from build123d import *

# Parameters (mm, degrees)
F1_DEPTH  = 85
F2_R      = 10
F4_DEPTH  = 6
F5_R      = 2
F6_W      = 7.7781745931
F6_H      = 15
F7_DEPTH  = 6
F8_R      = 2
F6_R      = 1.1
F9_DEPTH  = 1.5
F3_R      = 1.1
F10_DEPTH = 1.5
F11_W     = 18.7703792453
F11_H     = 83
F12_DEPTH = 8


with BuildPart() as f1:
    # F0 (on Top) → F1 (new body)
    with BuildSketch(Plane.XY):
        Polygon((-20, 20), (-14.5, 14.5), (-10.3851896226, 18.6148103774), (0, 18.6148103774), (10.3851896226, 18.6148103774), (14.5, 14.5), (20, 20), (12.470660899, 27.529339101), (0, 27.529339101), (-12.470660899, 27.529339101), align=None)
    extrude(amount=F1_DEPTH)

    # F2
    f2_edges = [f1.edges().sort_by_distance(p)[0] for p in [
        (-12.470661, 27.529339, 42.5),
        (12.470661, 27.529339, 42.5),
    ]]
    fillet(f2_edges, radius=F2_R)

    # F3 (on face) → F4 (cut)
    with BuildSketch(Plane(origin=(0, 0, 0), x_dir=(0.7071067812, 0.7071067812, 0), z_dir=(0.7071067812, -0.7071067812, 0))):
        Polygon((28.2842712475, 59.0200200677), (28.2842712475, 74.0199925453), (20.5060966544, 74.0199925453), (20.5060966544, 0), (20.6173848753, 0), (20.6173848753, 9.0200751125), (28.2842712475, 9.0200751125), (28.2842712475, 24.0200475901), (20.5802888017, 24.0200475901), (20.5802888017, 34.0200475901), (28.2842712475, 34.0200475901), (28.2842712475, 49.0200200677), (20.543192728, 49.0200200677), (20.543192728, 59.0200200677), align=None)
    extrude(amount=-F4_DEPTH, mode=Mode.SUBTRACT)

    # F5
    f5_edges = [f1.edges().sort_by_distance(p)[0] for p in [
        (17.87868, 22.12132, 74.019993),
        (17.87868, 22.12132, 49.02002),
        (17.87868, 22.12132, 24.020048),
        (17.699797, 22.300203, 0),
        (12.457372, 16.700013, 0),
        (12.431141, 16.673782, 24.020048),
        (12.404911, 16.647551, 49.02002),
        (17.699797, 22.300203, 85),
        (12.442595, 16.557405, 85),
        (17.87868, 22.12132, 59.02002),
        (12.404911, 16.647551, 59.02002),
        (17.87868, 22.12132, 34.020048),
        (12.431141, 16.673782, 34.020048),
        (17.87868, 22.12132, 9.020075),
        (12.457372, 16.700013, 9.020075),
        (-17.699797, 22.300203, 0),
        (-17.699797, 22.300203, 85),
        (-12.15536, 26.768134, 0),
        (0, 27.529339, 0),
        (12.15536, 26.768134, 0),
        (-12.442595, 16.557405, 0),
        (-12.15536, 26.768134, 85),
        (0, 27.529339, 85),
        (-12.442595, 16.557405, 85),
        (12.15536, 26.768134, 85),
        (12.442595, 16.557405, 74.019993),
    ]]
    fillet(f5_edges, radius=F5_R)

    # F6 (on face) → F7 (cut)
    with BuildSketch(Plane(origin=(0, 0, 0), x_dir=(0.7071067812, -0.7071067812, 0), z_dir=(-0.7071067812, -0.7071067812, 0))):
        with Locations((-24.3951839509, 17.5)):
            Rectangle(F6_W, F6_H)
        with Locations((-24.3951839509, 42.5)):
            Rectangle(F6_W, F6_H)
        with Locations((-24.3951839509, 67.5)):
            Rectangle(F6_W, F6_H)
    extrude(amount=-F7_DEPTH, mode=Mode.SUBTRACT)

    # F8
    f8_edges = [f1.edges().sort_by_distance(p)[0] for p in [
        (-17.87868, 22.12132, 35),
        (-17.87868, 22.12132, 50),
        (-17.87868, 22.12132, 60),
        (-17.87868, 22.12132, 75),
        (-12.442595, 16.557405, 75),
        (-12.442595, 16.557405, 60),
        (-12.442595, 16.557405, 50),
        (-12.442595, 16.557405, 35),
        (-12.442595, 16.557405, 25),
        (-12.442595, 16.557405, 10),
        (-17.87868, 22.12132, 10),
        (-17.87868, 22.12132, 25),
    ]]
    fillet(f8_edges, radius=F8_R)

    # F6 (on face) → F9 (join)
    with BuildSketch(Plane(origin=(0, 0, 0), x_dir=(0.7071067812, -0.7071067812, 0), z_dir=(-0.7071067812, -0.7071067812, 0))):
        with Locations((-24.3951839509, 5)):
            Circle(F6_R)
        with Locations((-24.3951839509, 30)):
            Circle(F6_R)
        with Locations((-24.3951839509, 55)):
            Circle(F6_R)
        with Locations((-24.3951839509, 80)):
            Circle(F6_R)
    extrude(amount=F9_DEPTH)

    # F3 (on face) → F10 (join)
    with BuildSketch(Plane(origin=(0, 0, 0), x_dir=(0.7071067812, 0.7071067812, 0), z_dir=(0.7071067812, -0.7071067812, 0))):
        with Locations((24.3951839509, 79.0199925453)):
            Circle(F3_R)
        with Locations((24.4336626312, 54.0200221575)):
            Circle(F3_R)
        with Locations((24.4721413114, 29.0200517697)):
            Circle(F3_R)
        with Locations((24.5106199916, 4.0200813819)):
            Circle(F3_R)
    extrude(amount=F10_DEPTH)

    # F11 (on face) → F12 (cut)
    with BuildSketch(Plane.XZ.offset(-18.6148103774)):
        with Locations((0, 42.5)):
            Rectangle(F11_W, F11_H)
    extrude(amount=-F12_DEPTH, mode=Mode.SUBTRACT)


solid = f1.part
Source: CAD feature listing. Evaluate the final solid. Frame: model axes, mm. A direction names the side the tool comes from. Round coordinates to 2 decimals unless told otherwise and drop trailing zeros. Order: outer loops, then holes, each group sorted by start corner. A loop starts at its lowest first (then second) coordinate and runs counter-clockwise, first axis right, second up. Notation, with made-up numbers: (-10.75, 26) -> (20.25, 26) arc R16 cw to (20.25, 34) -> close; hole circle Ø10 at (-13.75, 15.25). An arc over 180 degrees is marked (long way). Answer as CSV lines item,"result".
Item 1: Reachability of faces 1 (the face through (-12.84, 17.01, 84.43)), 2 (the face through (15, 19, 9.02)), 3 (the face through (-17.446, 21.748, 9.399)), 4 (the face through (-12.82, 16.99, 75.6)), 5 (the face through (-12, 17, 5)) from +Z, -Z, +X, -X, +Y, -Y: full face, straight path, thin tool, end or side. Return the list, or none.
A:
face 1,"+Z, -Y"
face 2,"+X, -Y"
face 3,"-X"
face 4,"-Y"
face 5,"+Z, -Z, -Y"
Item 2: Section A-A, the plane z = 44. Return loops of the section in (x, y).
A:
outline,"(-15.76, 24.24) -> (-10.26, 18.74) -> (-10.39, 18.61) -> (-9.39, 18.61) -> (-9.39, 26.61) -> (9.39, 26.61) -> (9.39, 18.61) -> (10.39, 18.61) -> (10.26, 18.74) -> (15.76, 24.24) -> (15.4, 24.6) arc R10 ccw to (8.33, 27.53) -> (-8.33, 27.53) arc R10 ccw to (-15.4, 24.6) -> close"
Item 3: Pull-direction query (X, two-part tool) for faces 6 (the face through (-17.446, 21.748, 75.601)), 7 (the face through (12.827, 17.129, 33.45)), 8 (the face through (0, 27.529, 42)); classes: pulls with the +X half, pulls with the -X half, needs draft (parallel to the pull), parting line crosses it, or undercut.
A:
face 6,"pulls with the -X half"
face 7,"undercut"
face 8,"needs draft"
Item 4: Section B-B, the plane x = -7.5. Return loops of the section in (y, z), plus the area to 3 significant figures.
A:
outline,"(18.61, 0) -> (25.53, 0) arc R2 ccw to (27.53, 2) -> (27.53, 83) arc R2 ccw to (25.53, 85) -> (18.61, 85) -> (18.61, 84) -> (26.61, 84) -> (26.61, 1) -> (18.61, 1) -> close"
area,"92.0 mm²"
Item 5: Line query: L1, parallel to X at y = 18.75, z = 13; L2, parallel to Z at x = 15, y = 16.25; L3, parallel to Z at x = -6, y = 23. Output: solid intervals per line, ascending.
A:
L1,"-10.26 to -9.39, 9.39 to 10.26"
L2,"0.07 to 8.95, 24.08 to 33.96, 49.07 to 58.97, 74.06 to 84.96"
L3,"0 to 1, 84 to 85"
Item 6: Pin query (flat end, axial travel): pin 1 Ø4 at (x, y) = (2, 18.5) entering from +Z; pin 2 Ø4 at (y, z) = (24, 44.5) entering from +X; pin 3 Ø5.5 at (x, z) = (1.5, 62) entering from -Y; pin 4 Ø21 at (x, z) = (1.5, 54) entering from -Y. Return the tip coordinate at first contact, or that it passes through.
A:
pin 1,"z = 85"
pin 2,"x = 15.76"
pin 3,"y = 26.61"
pin 4,"y = 17.05"
